Work out the finished part from the listing and answer in its coordinate system (mm). Face numbers are marked on the shaded views. A direction names the side the tool comes from. Round coordinates to 2 decimals unless told otherwise and drop trailing zeros. Order: outer loops, then holes, each group sorted by start corner. A loop starts at its lowest first (then second) coordinate and runs counter-clockwise, first axis right, second up.
Autodesk Inventor part; units mm, degrees
ref_plane "YZ Plane" through (0, 0, 0) normal (1, 0, 0) x (0, 1, 0)
ref_plane "XZ Plane" through (0, 0, 0) normal (0, 1, 0) x (-1, 0, 0)
ref_plane "XY Plane" through (0, 0, 0) normal (0, 0, 1) x (1, 0, 0)
sketch "Sketch1" plane through (0, 0, 0) normal (0, 0, 1) x (1, 0, 0)
  line L0 (0, 0) -> (124, 0)
  line L1 (124, 0) -> (124, 124)
  line L2 (124, 124) -> (0, 124)
  line L3 (0, 124) -> (0, 0)
  circle A0 centre (62, 19.5) radius 2.5
  point P0 (62, 0)
  dimension "d0" = 124
  dimension "d1" = 124
  dimension "d2" = 5
  dimension "d3" = 19.5
extrude "Extrusion1" add sketch "Sketch1" along normal blind 10
sketch "Sketch2" plane through (0, 0, 10) normal (0, 0, 1) x (1, 0, 0)
  line L0 (0, 124) -> (0, 0)
  line L1 (0, 82) -> (-10, 82)
  line L2 (-10, 82) -> (-10, 42)
  line L3 (-10, 42) -> (0, 42)
  line L4 (0, 42) -> (0, 82)
  circle A0 centre (-5, 62) radius 2.5
  point P0 (-10, 62)
  point P1 (0, 62)
  point P2 (-5, 82)
  dimension "d8" = 10
  dimension "d9" = 40
  dimension "d10" = 5
extrude "Extrusion2" add sketch "Sketch2" against normal blind 5
sketch "Sketch3" plane through (0, 0, 10) normal (0, 0, 1) x (1, 0, 0)
  line L0 (124, 0) -> (124, 124)
  line L1 (124, 41) -> (112, 41)
  line L2 (112, 41) -> (112, 83)
  line L3 (112, 83) -> (124, 83)
  line L4 (124, 83) -> (124, 41)
  point P0 (0, 0)
  point P1 (112, 62)
  point P2 (124, 62)
  dimension "d13" = 12
  dimension "d14" = 42
extrude "Extrusion3" cut sketch "Sketch3" against normal blind 6
sketch "Sketch4" plane through (0, 0, 4) normal (0, 0, 1) x (1, 0, 0)
  line L0 (124, 41) -> (112, 41) construction
  line L1 (124, 83) -> (124, 41) construction
  line L2 (112, 83) -> (124, 83) construction
  line L3 (112, 41) -> (112, 83) construction
  circle A0 centre (119, 62) radius 2.5
  point P0 (0, 0)
  point P1 (124, 62)
  point P2 (118, 41)
  dimension "d17" = 5
  dimension "d28" = 5
extrude "Extrusion4" cut sketch "Sketch4" against normal through all
sketch "Sketch5" plane through (0, 0, 10) normal (0, 0, 1) x (1, 0, 0)
  line L0 (41, 124) -> (83, 124)
  line L1 (83, 124) -> (83, 112)
  line L2 (83, 112) -> (41, 112)
  line L3 (41, 112) -> (41, 124)
  line L4 (124, 124) -> (0, 124)
  point P0 (0, 0)
  point P1 (62, 112)
  point P2 (62, 124)
  dimension "d20" = 42
  dimension "d21" = 12
extrude "Extrusion5" cut sketch "Sketch5" against normal blind 6
sketch "Sketch6" plane through (0, 0, 4) normal (0, 0, 1) x (1, 0, 0)
  circle A0 centre (62, 119) radius 2.5
  line L0 (41, 124) -> (83, 124) construction
  line L1 (41, 112) -> (41, 124) construction
  line L2 (83, 112) -> (41, 112) construction
  line L3 (83, 124) -> (83, 112) construction
  point P0 (0, 0)
  point P1 (83, 118)
  point P2 (62, 124)
  dimension "d24" = 5
  dimension "d27" = 5
extrude "Extrusion6" cut sketch "Sketch6" against normal through all
properties part number "TA002" material "ABS Plastic"
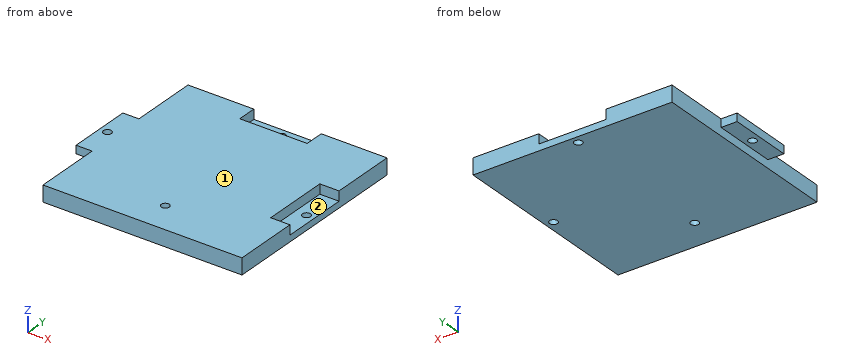
Item 1: Find section A-A (x = 62). Write down the section's boundary in (y, z).
Item 2: A tool of negligible diameter and unlimited length cuts with its end or side. For the marked faces 1 and 2, from which of +Z, -Z, +X, -X, +Y, -Y can it reach the whole face along a straight path? Write none if from no direction.
Item 3: Given pin 1 (8 mm diameter, centred on x = 119, y = 62, fed in from +Z); pin 2 (3 mm diameter, centred on y = 118.5, z = 8.5, fed in from -X); pin 3 (1.8 mm diameter, centred on y = 61, z = 7.5, fed in from +X), each flat-ended and moving along its own axis, determine where each tip first touches the part or whether it passes through.
Item 4: Find section B-B (y = 19.5). Write down the section's boundary in (x, z).
Item 5: Find the intervals of material crossed by line 1 along Y through (x, z) = (62, 3); line 2 along Y through (x, z) = (-5, 7.8); line 3 along X through (y, z) = (41.5, 8), in increasing order.
Item 6: Find section C-C (x = 119). Write down the section's boundary in (y, z), plus the area to 3 significant figures.
Item 7: Find section D-D (z = 6.75). Write down the section's boundary in (x, y), plus the area to 3 significant figures.
Model answer:
1. outline: (0, 0) - (17, 0) - (17, 10) - (0, 10) - close; (22, 0) - (116.5, 0) - (116.5, 4) - (112, 4) - (112, 10) - (22, 10) - close; (121.5, 0) - (124, 0) - (124, 4) - (121.5, 4) - close
2. face 1: +Z, +X, -X, +Y, -Y
2. face 2: +Z, +X
3. pin 1: stops at z = 4
3. pin 2: stops at x = 0
3. pin 3: stops at x = 112
4. outline: (0, 0) - (59.5, 0) - (59.5, 10) - (0, 10) - close; (64.5, 0) - (124, 0) - (124, 10) - (64.5, 10) - close
5. line 1: y = 0 to 17, 22 to 116.5, 121.5 to 124
5. line 2: y = 42 to 59.5, 64.5 to 82
5. line 3: x = 0 to 112
6. outline: (0, 0) - (59.5, 0) - (59.5, 4) - (41, 4) - (41, 10) - (0, 10) - close; (64.5, 0) - (124, 0) - (124, 10) - (83, 10) - (83, 4) - (64.5, 4) - close
6. area: 968 mm2
7. outline: (-10, 42) - (0, 42) - (0, 0) - (124, 0) - (124, 41) - (112, 41) - (112, 83) - (124, 83) - (124, 124) - (83, 124) - (83, 112) - (41, 112) - (41, 124) - (0, 124) - (0, 82) - (-10, 82) - close; hole circle Ø5 at (-5, 62); hole circle Ø5 at (62, 19.5)
7. area: 14,700 mm2
